Here's the drawing with two shaded views (mm, measured from the low corner). I have some questions. Round coordinates to 2 decimals unless told otherwise and drop trailing zeros. Loops run counter-clockwise (first coordinate to the right, second up) from the corner with the lowest first, then second, coordinate; pieces in that order, holes last.
(1) I want a section at B-B on x = 14.5. Write out the boundary of the cut face in (y, z).
(2) I want a section at A-A on y = 211. Write out the boundary of the cut face in (x, z).
(3) If I drill on line 1 along X through (y, z) = (125, 5); line 2 along Y through (x, z) = (75, 3.5); line 3 along X through (y, z) = (187, 4), over which ranges is the centre line in solid material (lowest first)?
(4) Will these pins go through, and if not, where does the flat tip stop? pin 1 Ø5 at (x, z) = (144.5, 5) entering from -Y; pin 2 Ø5 at (x, z) = (42.5, 3) entering from +Y; pin 3 Ø5 at (x, z) = (27, 2.5) entering from -Y.
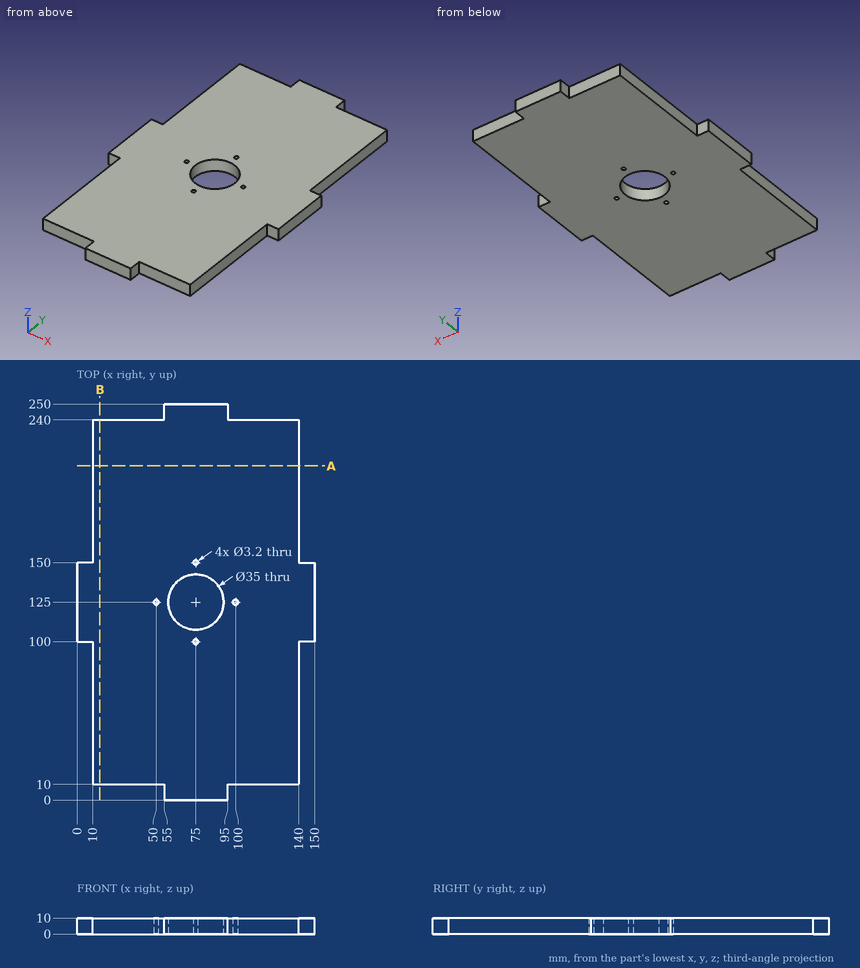
Filled sheet:
1. outline: (10, 0) - (240, 0) - (240, 10) - (10, 10) - close
2. outline: (10, 0) - (140, 0) - (140, 10) - (10, 10) - close
3. line 1: x = 0 to 48.4, 51.6 to 57.5, 92.5 to 98.4, 101.6 to 150
3. line 2: y = 0 to 98.4, 101.6 to 107.5, 142.5 to 148.4, 151.6 to 250
3. line 3: x = 10 to 140
4. pin 1: stops at y = 100
4. pin 2: stops at y = 240
4. pin 3: stops at y = 10
